```python
from build123d import *

# Parameters (mm, degrees)
BOSS_EXTRUDE1_DEPTH     = 12
SKETCH2_R               = 3.15
CUT_EXTRUDE1_DEPTH      = 7
CUT_EXTRUDE1_DEPTH_BACK = 7


with BuildPart() as part:
    # Sketch1 → Boss-Extrude1 (new body)
    with BuildSketch(Plane.XY):
        with BuildLine():
            Line((0, 6), (12, 6))
            Line((12, 6), (12, 2.552710574))
            Line((12, 2.552710574), (2.091331807, 2.552710574))
            ThreePointArc((2.091331807, 2.552710574), (-3.3, 0), (2.091331807, -2.552710574))
            Line((2.091331807, -2.552710574), (12, -2.552710574))
            Line((12, -2.552710574), (12, -6))
            Line((12, -6), (0, -6))
            ThreePointArc((0, -6), (-6, 0), (0, 6))
        make_face()
    extrude(amount=BOSS_EXTRUDE1_DEPTH)

    # Sketch2 → Cut-Extrude1 (cut, two sides)
    with BuildSketch(Plane(origin=(0, 0, 0), x_dir=(1, 0, 0), z_dir=(0, 1, 0))) as cut_extrude1_sk:
        with Locations((6, -6)):
            Circle(SKETCH2_R)
    extrude(amount=CUT_EXTRUDE1_DEPTH, mode=Mode.SUBTRACT)
    extrude(cut_extrude1_sk.sketch, amount=-CUT_EXTRUDE1_DEPTH_BACK, mode=Mode.SUBTRACT)


solid = part.part
```
Read the model definition and answer for the solid it produces. Units are mm, in the model's axes. A direction names the side the tool comes from. Give positions to 0.01 mm unless a question says otherwise; leave off trailing zeros. Write each loop counter-clockwise with the first axis right and the second up, starting at its lowest first coordinate (ties: lowest second). Pieces come first, ordered by that corner, then holes. Notation, with made-up numbers: (-32.5, 25) -> (24.5, 25) arc R37 cw to (24.5, 62) -> close; hole circle Ø3 at (-40, -2). An arc over 180 degrees is marked (long way). Answer as a JSON object with one key per item and string values.
1) A tool of negligible diameter and unlimited length cuts with its end or side. For faces 4 (the flat face through (9.3, 2.553, 5.9)), 5 (the cylindrical face through (-6, 0, 6)), from which of +Z, -Z, +X, -X, +Y, -Y can it reach the whole face along a straight path? Write none if from no direction.
Findings below:
{"face 4": "+Z, -Z, +X", "face 5": "+Z, -Z, -X"}
2) A flat-ended cylindrical pin translates along its axis: pin 1 Ø2 at (y, z) = (4.5, 5.5) entering from -X. Find the tip coordinate at first contact, or state that the pin passes through.
Findings below:
{"pin 1": "stops at x = -4.87"}
3) Section D-D on z = 10.5 is taken. Write down the section's boundary in (x, y).
Findings below:
{"outline": "(0, -6) -> (12, -6) -> (12, -2.55) -> (2.09, -2.55) arc R3.3 cw (long way) to (2.09, 2.55) -> (12, 2.55) -> (12, 6) -> (0, 6) arc R6 ccw to start"}
4) Section C-C on x = 2.5 is taken. Write down the section's boundary in (y, z).
Findings below:
{"outline": "(-6, 0) -> (-2.55, 0) -> (-2.55, 12) -> (-6, 12) -> close; (2.55, 0) -> (6, 0) -> (6, 12) -> (2.55, 12) -> close"}
5) Section B-B on z = 6 is taken. Write down the section's boundary in (x, y), then the cut area to 3 significant figures.
Findings below:
{"outline": "(0, -6) -> (2.85, -6) -> (2.85, -2.55) -> (2.09, -2.55) arc R3.3 cw (long way) to (2.09, 2.55) -> (2.85, 2.55) -> (2.85, 6) -> (0, 6) arc R6 ccw to start; (9.15, -6) -> (12, -6) -> (12, -2.55) -> (9.15, -2.55) -> close; (9.15, 2.55) -> (12, 2.55) -> (12, 6) -> (9.15, 6) -> close", "area": "76.6 mm^2"}
6) Section A-A on x = 6 is taken. Write down the section's boundary in (y, z).
Findings below:
{"outline": "(-6, 0) -> (-2.55, 0) -> (-2.55, 2.85) -> (-6, 2.85) -> close; (-6, 9.15) -> (-2.55, 9.15) -> (-2.55, 12) -> (-6, 12) -> close; (2.55, 0) -> (6, 0) -> (6, 2.85) -> (2.55, 2.85) -> close; (2.55, 9.15) -> (6, 9.15) -> (6, 12) -> (2.55, 12) -> close"}
7) Straight lines are drawn through the part: probe 1 along Y at (x, z) = (2.5, 9.25); probe 2 along Y at (x, z) = (0, 7); probe 3 along Z at (x, y) = (6, -3.7). For each, find the intervals that lie inside material, in ascending order. Write a range as from..to.
Findings below:
{"probe 1": "y = -6..-2.55, 2.55..6", "probe 2": "y = -6..-3.3, 3.3..6", "probe 3": "z = 0..2.85, 9.15..12"}
8) For a pull along X with two mould halves and no side action, classify faces 1 (the flat face through (3, -3, 12)), 2 (the flat face through (12, -4, 6)), 3 (the cylindrical face through (9.005, 4.252, 5.054)) as pulls with the +X half, pulls with the -X half, needs draft (parallel to the pull), parting line crosses it, or undercut.
Findings below:
{"face 1": "needs draft", "face 2": "pulls with the +X half", "face 3": "undercut"}
